Autodesk Inventor part; units mm, degrees
ref_plane "Work Plane1" through (6, 0, 0) normal (0, -0.5, -0.866) x (1, 0, 0)
ref_plane "YZ Plane" through (0, 0, 0) normal (1, 0, 0) x (0, 1, 0)
ref_plane "XZ Plane" through (0, 0, 0) normal (0, 1, 0) x (-1, 0, 0)
sketch "Skizze1" plane through (0, 0, 0) normal (0, 0, 1) x (1, 0, 0)
  line L0 (0.7217, 0) -> (8.1667, 0)
  line L1 (12, 1.4434) -> (12, 2.5)
  line L2 (12, 2.5) -> (0, 2.5)
  line L3 (12, 1.4434) -> (9, 1.4434)
  line L4 (9, 1.4434) -> (8.1667, 0)
  line L5 (0, 1.25) -> (0.7217, 0)
  line L6 (0, -0.5) -> (0, 3)
  line L7 (0, 1.25) -> (0, 2.5)
  point P0 (0, 0)
  dimension "d0" = 3
  dimension "d1" = 60
  dimension "d2" = 5
  dimension "d3" = 2.8868
  dimension "d4" = 12
  dimension "d5" = 60
  dimension "d7" = 2.5
revolve "Körper" add sketch "Skizze1" angle 360 about axis through (0.7217, 0, 0) along (1, 0, 0)
sketch "Skizze2" plane through (12, 0, 0) normal (1, 0, 0) x (0, 0, -1)
  circle A0 centre (0, 0) radius 1.4434
  circle A1 centre (0, 0) radius 2.5
  line L0 (1.4434, 0) -> (0.7217, -1.25)
  line L1 (0.7217, -1.25) -> (-0.7217, -1.25)
  line L2 (-0.7217, -1.25) -> (-1.4434, 0)
  line L3 (-1.4434, 0) -> (-0.7217, 1.25)
  line L4 (-0.7217, 1.25) -> (0.7217, 1.25)
  line L5 (0.7217, 1.25) -> (1.4434, 0)
extrude "Loch" add sketch "Skizze2" against normal blind 3 contours L5 A0 | A0 L0 | L4 A0 | A0 L1 | L3 A0 | A0 L2
chamfer "Fase1" distance 1.25 angle 45 1 edges at (0, -2.5, 0) measured on face at (0, 2.0591, -0.1994)
thread "Gewinde"
chamfer "Fase2" distance 0.4908 angle 45 1 edges at (12, -2.5, 0) measured on face at (4.833, 2.4919, -0.2012)
ref_plane "Work Plane1" through (6, 0, 0) normal (0, -0.5, -0.866) x (1, 0, 0)
equation "\"d0\" = INTI"
equation "\"d2\" = NND"
equation "\"d3\" = 1.1547 * SW"
equation "\"d4\" = NLG"
equation "\"d5\" = 0.5 * ANG"
equation "\"d7\" = SPD"
equation "\"d8\" = INTI"
equation "\"d10\" = -0.5 * SPD + 0.5 * NND"
equation "\"d11\" = FAWI"
equation "\"d33\" = -0.5 * SPD + 0.5 * NND"
equation "\"d14\" = NLG"
equation "\"d12\" = -0.5 * GD1 + 0.5 * NND"
equation "\"d13\" = FAWI"
equation "\"d34\" = -0.5 * GD1 + 0.5 * NND"
equation "\"NND\" = 5"
equation "\"NLG\" = 12"
equation "\"INTI\" = 3"
equation "\"FAWI\" = 45deg"
equation "\"SW\" = 2.5"
equation "\"GD1\" = THREADDIA - 1.2269 * PTC"
equation "\"ANG\" = 120deg"
equation "\"FAWI1\" = 45deg"
equation "\"SPD\" = 2.5"
equation "\"GUL\" = 0.61345 * PTC"
equation "\"TOA\" = 30deg"
equation "\"THREADDIA\" = 5"
equation "\"PTC\" = 0.8"
equation "\"GAL\" = 0.61345 * PTC"
equation "\"E0\" = 1.155 * SW"
properties part number "ISO 4029 - M5 x 12" material "Edelstahl, 440C"
Can you work these out from the model? Positions are in its coordinate system, mm. Coordinates: 2 decimals unless noted, no trailing zeros. Write each loop counter-clockwise with the first axis right and the second up, starting at its lowest first coordinate (ties: lowest second). Pieces come first, ordered by that corner, then holes. Notation, with made-up numbers: M -38,-7.75 L -9,-7.75 A26 ccw -9,17.25 Z; hole C 74.25,9.5 d3. An arc over 180 degrees is marked long. Answer as CSV lines item,"result".
Item 1: I'm going to push flat-ended pins straight in: P1, Ø2, axis at y = 2, z = -1.5, coming from the -X side; P2, Ø1, axis at y = -0.5, z = -0.5, coming from the +X side. Where does each tip first touch, or does it pass through?
Geometry results:
P1,"stops at x = 0.25"
P2,"stops at x = 8.86"
Item 2: We'd pull the mould along Y, two halves only. Please class faces 1 (the cylindrical face through (6.31, -0.54, 2.44)), 2 (the conical face through (0.596, -0.047, 0.212)), 3 (the conical face through (8.311, 0.239, 0.075)): +Y half, -Y half, draft (parallel to the pull), parting line (faces both ways), or undercut.
Geometry results:
face 1,"parting line"
face 2,"undercut"
face 3,"undercut"
Item 3: Imagine slicing it at B-B on x = 8.5. List the corners of the cut face in (y, z) for me.
Geometry results:
outline,"C 0,0 d5; hole C 0,0 d1.15"
Item 4: Imagine slicing it at A-A on x = 5.5. List the corners of the cut face in (y, z) for me.
Geometry results:
outline,"C 0,0 d5"
Item 5: Please list where these lines run through material, in increasing order: line 1 along Y through (x, z) = (10, 0.5); line 2 along Y through (x, z) = (9.75, -1.25); line 3 along Y through (x, z) = (5.5, -0.1).
Geometry results:
line 1,"y = -2.45 to -1.25, 1.25 to 2.45"
line 2,"y = -2.17 to -0.33, 0.33 to 2.17"
line 3,"y = -2.5 to 2.5"
